The model under review builds one solid part; all positions refer to its coordinate system, in mm. A direction names the side the tool comes from. Give positions to 0.01 mm unless a question says otherwise; leave off trailing zeros. Use CSV: the item, a comma, the result in double quotes.
```python
from build123d import *

# Parameters (mm, degrees)
BOSS_EXTRUDE1_DEPTH      = 2
F_4_0MM_DOWEL_HOLE1_D    = 4
M3_CLEARANCE_HOLE1_D     = 3.4
M3_CLEARANCE_HOLE1_DEPTH = 10
M3_CLEARANCE_HOLE1_TIP   = 1.021463052
M2_CLEARANCE_HOLE1_D     = 2.4
M2_CLEARANCE_HOLE1_DEPTH = 10
M2_CLEARANCE_HOLE1_TIP   = 0.721032743


with BuildPart() as part:
    # Sketch1 → Boss-Extrude1 (new body)
    with BuildSketch(Plane(origin=(0, 0, 0), x_dir=(1, 0, 0), z_dir=(0, 1, 0))):
        Polygon((-53.970588235, 35.110294118), (-41.470588235, 35.110294118), (-41.470588235, 47.610294118), (23.529411765, 47.610294118), (23.529411765, 35.110294118), (36.029411765, 35.110294118), (36.029411765, -29.889705882), (23.529411765, -29.889705882), (23.529411765, -42.389705882), (-41.470588235, -42.389705882), (-41.470588235, -29.889705882), (-53.970588235, -29.889705882), align=None)
    extrude(amount=BOSS_EXTRUDE1_DEPTH)

    # Ø4.0mm Dowel Hole1 (through all)
    with Locations(Plane(origin=(0, 2, 0), x_dir=(1, 0, 0), z_dir=(0, 1, 0))):
        with Locations((-43.970588235, 25.110294118), (26.029411765, 25.110294118), (-43.970588235, -19.889705882), (26.029411765, -19.889705882)):
            Hole(F_4_0MM_DOWEL_HOLE1_D / 2)

    # M3 Clearance Hole1
    with Locations(Plane(origin=(0, 2, 0), x_dir=(1, 0, 0), z_dir=(0, 1, 0))):
        with Locations((-37.970588235, -9.389705882), (-37.970588235, -32.389705882), (20.029411765, -32.389705882), (20.029411765, -9.389705882)):
            Hole(M3_CLEARANCE_HOLE1_D / 2, depth=M3_CLEARANCE_HOLE1_DEPTH)
            with Locations((0, 0, -(M3_CLEARANCE_HOLE1_DEPTH + M3_CLEARANCE_HOLE1_TIP / 2))):  # 118° drill point
                Cone(0, M3_CLEARANCE_HOLE1_D / 2, M3_CLEARANCE_HOLE1_TIP, mode=Mode.SUBTRACT)

    # M2 Clearance Hole1
    with Locations(Plane(origin=(0, 2, 0), x_dir=(1, 0, 0), z_dir=(0, 1, 0))):
        with Locations((-31.470588235, -39.889705882), (-31.470588235, -6.889705882), (13.529411765, -39.889705882), (13.529411765, -6.889705882)):
            Hole(M2_CLEARANCE_HOLE1_D / 2, depth=M2_CLEARANCE_HOLE1_DEPTH)
            with Locations((0, 0, -(M2_CLEARANCE_HOLE1_DEPTH + M2_CLEARANCE_HOLE1_TIP / 2))):  # 118° drill point
                Cone(0, M2_CLEARANCE_HOLE1_D / 2, M2_CLEARANCE_HOLE1_TIP, mode=Mode.SUBTRACT)


solid = part.part
```
Item 1: Wall thickness on L1, parallel to X at y = 1.2, z = 20; L2, parallel to Z at x = 26.5, y = 0.6; L3, parallel to X at y = 0.9, z = 21: over which ranges is each line inside the solid? List them lowest first.
Results list:
L1,"x = -53.97 to -45.97, -41.97 to 24.03, 28.03 to 36.03"
L2,"z = -35.11 to -27.05, -23.17 to 17.95, 21.83 to 29.89"
L3,"x = -53.97 to -45.63, -42.31 to 24.37, 27.69 to 36.03"
Item 2: Tool access review of faces 1 (the face through (-48, 1, 29.89)), 2 (the face through (23.529, 1, -41)), 3 (the face through (30, 1, 29.89)): name each direction out of +Z, -Z, +X, -X, +Y, -Y from which nothing blocks a thin tool from reaching the whole face with its end or side.
Results list:
face 1,"+Z, -X, +Y, -Y"
face 2,"-Z, +X, +Y, -Y"
face 3,"+Z, +X, +Y, -Y"
Item 3: Mouldability with a two-part tool opening along Z and no side actions: class faces 4 (the face through (27.617, 0.986, 21.107)), 5 (the face through (-9, 1, -47.61)), 6 (the face through (-41.471, 1, -41)) as pulls with the +Z half, pulls with the -Z half, needs draft (parallel to the pull), parting line crosses it, or undercut.
Results list:
face 4,"undercut"
face 5,"pulls with the -Z half"
face 6,"needs draft"
Item 4: Clearance check with flat-ended pins moving along their axes: pin 1 (4 mm diameter, centred on x = 13.53, z = 6.89, fed in from +Y); pin 2 (3.5 mm diameter, centred on x = -43.97, z = -25.11, fed in from +Y); pin 3 (1 mm diameter, centred on x = 32, y = 1.5, fed in from +Z); pin 4 (1 mm diameter, centred on y = 1.5, z = -44.5, fed in from -X). State where each tip first meets the part, or that it passes through.
Results list:
pin 1,"stops at y = 2"
pin 2,"passes through"
pin 3,"stops at z = 29.89"
pin 4,"stops at x = -41.47"
Item 5: Take a section at A-A, the plane y = 1.55. State how many separate pieces and enclosed holes the cut face has, and give its area (3 significant figures).
Results list:
separate pieces,"1"
enclosed holes,"12"
area,"7,370 mm2"
